Build history of the part. All positions in model axes, mm. Face numbers are marked on the shaded views. A direction names the side the tool comes from. Round coordinates to 2 decimals unless told otherwise and drop trailing zeros. Write each loop counter-clockwise with the first axis right and the second up, starting at its lowest first coordinate (ties: lowest second). Pieces come first, ordered by that corner, then holes. Notation, with made-up numbers: (29, 69) - (54, 69) arc R29 ccw to (54, 97) - close; hole circle Ø3 at (0, -11). An arc over 180 degrees is marked (long way). Answer as a JSON object with one key per item and string values. Group by question number.
Item 1: Slice it at D-D, the plane y = -12.75. List the corners of the cut face in (x, z), then the cut area to 3 significant figures.
Item 2: Flat gauge pins, fed straight in: pin 1 (4 mm diameter, centred on x = 15.5, y = -12.75, fed in from +Z); pin 2 (3 mm diameter, centred on x = 23.5, z = 2, fed in from +Y); pin 3 (3 mm diameter, centred on y = -9.5, z = 5, fed in from -X). Where does each tip first touch, or does it go through?
Item 3: Which spindle directions (+Z, -Z, +X, -X, +Y, -Y) get a long thin tool onto all of the face, cutting with end or side? Do the marked faces 4, 5 and 6. Say none if no direction does.
Item 4: Slice it at B-B, the plane z = 4.8. List the corners of the cut face in (x, y).
Item 5: Slice it at A-A, the plane x = 0. List the corners of the cut face in (y, z), then the cut area to 3 significant figures.
Item 6: Probe line 1 (X direction, y = 18.25, z = 1.1); line 2 (Y direction, x = 15.5, z = 1.2); line 3 (X direction, y = -11.5, z = 0.5). List the from-to ranges inside material, lowest first. Write a range as from..to.
Item 7: Two-plate mould, pull along X, no slides. Class the marked faces 1, 2 and 3: +X half, -X half, draft (parallel to the pull), parting line (faces both ways), or undercut.
Item 8: Slice it at C-C, the plane y = 2.75. List the corners of the cut face in (x, z).
from build123d import *

# Parameters (mm, degrees)
ESBO_O1_R                = 1.75
ESBO_O1_R_2              = 11
RESSALTO_EXTRUS_O1_DEPTH = 6
FILETE1_R                = 5.5
ESBO_O2_R                = 3.5
CORTE_EXTRUS_O1_DEPTH    = 2


with BuildPart() as part:
    # Esboço1 → Ressalto-extrusão1 (new body)
    with BuildSketch(Plane.XY):
        with BuildLine():
            Line((-21, 23.75), (21, 23.75))
            Line((21, 23.75), (21, -9.75))
            Line((21, -9.75), (24.5, -9.75))
            ThreePointArc((24.5, -9.75), (31.5, -16.75), (24.5, -23.75))
            Line((24.5, -23.75), (21, -23.75))
            Line((21, -23.75), (-21, -23.75))
            Line((-21, -23.75), (-24.5, -23.75))
            ThreePointArc((-24.5, -23.75), (-31.5, -16.75), (-24.5, -9.75))
            Line((-24.5, -9.75), (-21, -9.75))
            Line((-21, -9.75), (-21, 23.75))
        make_face()
        with Locations((24.5, -16.75)):
            Circle(ESBO_O1_R, mode=Mode.SUBTRACT)
        with Locations((0, 2.75)):
            Circle(ESBO_O1_R_2, mode=Mode.SUBTRACT)
        with Locations((15.5, 18.25)):
            Circle(ESBO_O1_R, mode=Mode.SUBTRACT)
        with Locations((15.5, -12.75)):
            Circle(ESBO_O1_R, mode=Mode.SUBTRACT)
        with Locations((-15.5, 18.25)):
            Circle(ESBO_O1_R, mode=Mode.SUBTRACT)
        with Locations((-15.5, -12.75)):
            Circle(ESBO_O1_R, mode=Mode.SUBTRACT)
        with Locations((-24.5, -16.75)):
            Circle(ESBO_O1_R, mode=Mode.SUBTRACT)
    extrude(amount=RESSALTO_EXTRUS_O1_DEPTH)

    # Filete1
    filete1_edges = [part.edges().sort_by_distance(p)[0] for p in [
        (-21, 23.75, 3),
        (21, 23.75, 3),
    ]]
    fillet(filete1_edges, radius=FILETE1_R)

    # Esboço2 → Corte-extrusão1 (cut)
    with BuildSketch(Plane.XY.offset(6)):
        with Locations((-15.5, 18.25)):
            Circle(ESBO_O2_R)
        with Locations((15.5, 18.25)):
            Circle(ESBO_O2_R)
        with Locations((15.5, -12.75)):
            Circle(ESBO_O2_R)
        with Locations((-15.5, -12.75)):
            Circle(ESBO_O2_R)
    extrude(amount=-CORTE_EXTRUS_O1_DEPTH, mode=Mode.SUBTRACT)


solid = part.part
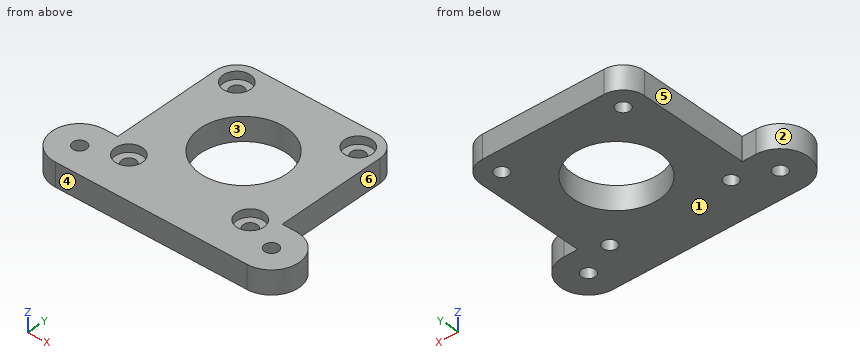
Geometry says:
{
 "1": {"outline": "(-30.24, 0) - (-17.25, 0) - (-17.25, 4) - (-19, 4) - (-19, 6) - (-30.24, 6) - close; (-13.75, 0) - (13.75, 0) - (13.75, 4) - (12, 4) - (12, 6) - (-12, 6) - (-12, 4) - (-13.75, 4) - close; (17.25, 0) - (30.24, 0) - (30.24, 6) - (19, 6) - (19, 4) - (17.25, 4) - close", "area": "307 mm^2"},
 "2": {"pin 1": "stops at z = 4", "pin 2": "stops at y = -9.75", "pin 3": "stops at x = -28.49"},
 "3": {"face 4": "+Z, -Z, +X, -X, -Y", "face 5": "+Z, -Z, -X, +Y", "face 6": "+Z, -Z, +X, +Y"},
 "4": {"outline": "(-24.5, -23.75) - (24.5, -23.75) arc R7 ccw to (24.5, -9.75) - (21, -9.75) - (21, 18.25) arc R5.5 ccw to (15.5, 23.75) - (-15.5, 23.75) arc R5.5 ccw to (-21, 18.25) - (-21, -9.75) - (-24.5, -9.75) arc R7 ccw to start; hole circle Ø3.5 at (-24.5, -16.75); hole circle Ø7 at (-15.5, -12.75); hole circle Ø7 at (-15.5, 18.25); hole circle Ø22 at (0, 2.75); hole circle Ø7 at (15.5, -12.75); hole circle Ø7 at (15.5, 18.25); hole circle Ø3.5 at (24.5, -16.75)"},
 "5": {"outline": "(-23.75, 0) - (-8.25, 0) - (-8.25, 6) - (-23.75, 6) - close; (13.75, 0) - (23.75, 0) - (23.75, 6) - (13.75, 6) - close", "area": "153 mm^2"},
 "6": {"line 1": "x = -21..-17.25, -13.75..13.75, 17.25..21", "line 2": "y = -23.75..-14.5, -11..16.5, 20..23.75", "line 3": "x = -29.13..-16.72, -14.28..14.28, 16.72..29.13"},
 "7": {"face 1": "draft", "face 2": "-X half", "face 3": "undercut"},
 "8": {"outline": "(-21, 0) - (-11, 0) - (-11, 6) - (-21, 6) - close; (11, 0) - (21, 0) - (21, 6) - (11, 6) - close"}
}
